Geometry: final body of the model. Coordinates: model frame, mm. A direction names the side the tool comes from. Round coordinates to 2 decimals unless told otherwise and drop trailing zeros. Write each loop counter-clockwise with the first axis right and the second up, starting at its lowest first coordinate (ties: lowest second). Pieces come first, ordered by that corner, then holes. Notation, with made-up numbers: M -1,-36 L 19,-36 A18 ccw 19,-13 Z; hole C 59,-11 d4. An arc over 180 degrees is marked long. Answer as CSV lines item,"result". Start each with the question number.
Q1. Section query C-C on z = 2. Output: boundary loops of the cut face in (x, y), and give its area (3 significant figures).
Q2. Ray query, probe 1 along Y at (x, z) = (2, 1.4); probe 2 along X at (y, z) = (-14, 2); probe 3 along X at (y, z) = (-17.25, 2.65). Return the intervals inside material, ascending.
Q3. Mould query, pull axis X, two halves, no side actions, for faces 1 (the cylindrical face through (16.25, -18.07, 1.95)), 2 (the flat face through (0, -12, 2)), 3 (the flat face through (35, -11, 0)). Classes: pulls with the +X half, pulls with the -X half, needs draft (parallel to the pull), parting line crosses it, or undercut.
Q4. Section query D-D on x = 35. Output: boundary loops of the cut face in (y, z).
Q5. Section query A-A on x = 2. Output: boundary loops of the cut face in (y, z), and give its area (3 significant figures).
Q6. Section query B-B on y = -6. Output: boundary loops of the cut face in (x, z), and give its area (3 significant figures).
Q7. First-contact query: pin 1 (0.8 mm diameter, centred on x = 15, z = 2, fed in from -Y); pin 2 (1.2 mm diameter, centred on y = -6.5, z = 2, fed in from +X). Flat tips, straight axial feed; report the tip coordinate or a pass-through.
Q8. Reachability of faces 4 (the cylindrical face through (0.5, -5.93, 2.03)), 5 (the flat face through (60, -17, 2)), 6 (the flat face through (55, -13, 2)) from +Z, -Z, +X, -X, +Y, -Y: full face, straight path, thin tool, end or side. Return the list, or none.
```python
from build123d import *

# Parameters (mm, degrees)
ESBO_O1_W                = 70
ESBO_O1_H                = 23
RESSALTO_EXTRUS_O1_DEPTH = 4
ESBO_O2_R                = 1.25
CORTE_EXTRUS_O1_DEPTH    = 10
ESBO_O3_R                = 1.25
CORTE_EXTRUS_O2_DEPTH    = 10
ESBO_O4_R                = 1.5
CORTE_EXTRUS_O3_DEPTH    = 10


with BuildPart() as part:
    # Esboço1 → Ressalto-extrusão1 (new body)
    with BuildSketch(Plane.XY):
        with Locations((35, -11.5)):
            Rectangle(ESBO_O1_W, ESBO_O1_H)
    extrude(amount=RESSALTO_EXTRUS_O1_DEPTH)

    # Esboço2 → Corte-extrusão1 (cut)
    with BuildSketch(Plane(origin=(70, 0, 0), x_dir=(0, 0, -1), z_dir=(1, 0, 0))):
        with Locations((-2, -6)):
            Circle(ESBO_O2_R)
        with Locations((-2, -17)):
            Circle(ESBO_O2_R)
    extrude(amount=-CORTE_EXTRUS_O1_DEPTH, mode=Mode.SUBTRACT)

    # Esboço3 → Corte-extrusão2 (cut)
    with BuildSketch(Plane(origin=(0, -23, 0), x_dir=(-1, 0, 0), z_dir=(0, -1, 0))):
        with Locations((-15, -2)):
            Circle(ESBO_O3_R)
        with Locations((-35, -2)):
            Circle(ESBO_O3_R)
        with Locations((-55, -2)):
            Circle(ESBO_O3_R)
    extrude(amount=-CORTE_EXTRUS_O2_DEPTH, mode=Mode.SUBTRACT)

    # Esboço4 → Corte-extrusão3 (cut)
    with BuildSketch(Plane.XY.offset(4)):
        with Locations((2, -6)):
            Circle(ESBO_O4_R)
        with Locations((2, -17)):
            Circle(ESBO_O4_R)
    extrude(amount=-CORTE_EXTRUS_O3_DEPTH, mode=Mode.SUBTRACT)


solid = part.part
```
Entries:
1,outline,"M 0,-23 L 13.75,-23 L 13.75,-13 L 16.25,-13 L 16.25,-23 L 33.75,-23 L 33.75,-13 L 36.25,-13 L 36.25,-23 L 53.75,-23 L 53.75,-13 L 56.25,-13 L 56.25,-23 L 70,-23 L 70,-18.25 L 60,-18.25 L 60,-15.75 L 70,-15.75 L 70,-7.25 L 60,-7.25 L 60,-4.75 L 70,-4.75 L 70,0 L 0,0 Z; hole C 2,-17 d3; hole C 2,-6 d3"
1,area,"1,470 mm^2"
2,probe 1,"y = -23 to -18.5, -15.5 to -7.5, -4.5 to 0"
2,probe 2,"x = 0 to 13.75, 16.25 to 33.75, 36.25 to 53.75, 56.25 to 70"
2,probe 3,"x = 0 to 0.52, 3.48 to 13.93, 16.07 to 33.93, 36.07 to 53.93, 56.07 to 60"
3,face 1,"undercut"
3,face 2,"pulls with the -X half"
3,face 3,"needs draft"
4,outline,"M -23,0 L 0,0 L 0,4 L -23,4 L -23,3.25 L -13,3.25 L -13,0.75 L -23,0.75 Z"
5,outline,"M -23,0 L -18.5,0 L -18.5,4 L -23,4 Z; M -15.5,0 L -7.5,0 L -7.5,4 L -15.5,4 Z; M -4.5,0 L 0,0 L 0,4 L -4.5,4 Z"
5,area,"68.0 mm^2"
6,outline,"M 0,0 L 0.5,0 L 0.5,4 L 0,4 Z; M 3.5,0 L 70,0 L 70,0.75 L 60,0.75 L 60,3.25 L 70,3.25 L 70,4 L 3.5,4 Z"
6,area,"243 mm^2"
7,pin 1,"stops at y = -13"
7,pin 2,"stops at x = 60"
8,face 4,"+Z, -Z"
8,face 5,"+X"
8,face 6,"-Y"
